Could you check a few things on this model? Use its own coordinates, in mm. Face numbers are marked on the shaded views. A direction names the side the tool comes from. Round coordinates to 2 decimals unless told otherwise and drop trailing zeros. Loops run counter-clockwise (first coordinate to the right, second up) from the corner with the lowest first, then second, coordinate; pieces in that order, holes last. Notation, with made-up numbers: (15.5, 25) - (50.5, 25) arc R26 ccw to (50.5, 43) - close; hole circle Ø6 at (0.25, 85). An arc over 180 degrees is marked (long way). Answer as CSV lines item,"result". Start each with the question number.
1) We'd pull the mould along Y, two halves only. Please class the marked faces 6, 7 and 8: pulls with the +Y half, pulls with the -Y half, needs draft (parallel to the pull), parting line crosses it, or undercut.
2) Suppose I cut it at B-B, the plane z = -155.5. Write out the boundary of the cut face in (x, y).
3) Suppose I cut it at D-D, the plane y = 74. Write out the boundary of the cut face in (x, z).
4) Suppose I cut it at A-A, the plane y = 41.5. Write out the boundary of the cut face in (x, z), then the cut area to 3 significant figures.
5) Please list where these lines run through material, in increasing order: line 1 along Z through (x, y) = (13.25, 49); line 2 along Z through (x, y) = (1.5, 51); line 3 along Z through (x, y) = (18, 42).
6) I'm going to push flat-ended pins straight in: pin 1 Ø1 at (x, y) = (7.5, 61.5) entering from -Z; pin 2 Ø10 at (x, y) = (7, 14.5) entering from +Z; pin 3 Ø2 at (x, z) = (14, -10.5) entering from +Y. Where does each tip first touch, or does it pass through?
7) Suppose I cut it at C-C, the plane y = 24. Write out the boundary of the cut face in (x, z), then the cut area to 3 significant figures.
8) Which directions (+Z, -Z, +X, -X, +Y, -Y) give clear straight access to the entire face, cutting with the end or side of a thin tool? Please do the marked faces 1, 2, 3, 4 and 5.
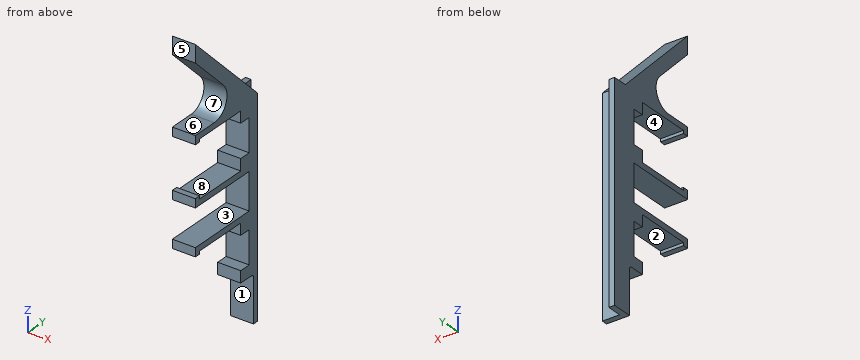
```python
from build123d import *

# Parameters (mm, degrees)
SKETCH1_W           = 5
SKETCH1_H           = 5
SKETCH1_W_2         = 35
BOSS_EXTRUDE2_DEPTH = 20
FILLET1_R           = 15
FILLET2_R           = 2
BOSS_EXTRUDE3_DEPTH = 12.7


with BuildPart() as part:
    # Sketch1 → Boss-Extrude2 (new body)
    with BuildSketch(Plane(origin=(0, 0, 0), x_dir=(0, 0, -1), z_dir=(1, 0, 0))):
        Polygon((-5, 53.5), (-5, 68.5), (-78.5, -5), (-63.5, -5), align=None)
        Polygon((69.5, 68.5), (-5, 68.5), (-5, 53.5), (-5, -5), (2.5, -5), (2.5, 0), (0, 0), (0, 48.5), (10, 48.5), (10, 58.5), (38.5, 58.5), (38.5, 48.5), (48.5, 48.5), (48.5, 0), (53.5, 0), (53.5, 58.5), (69.5, 58.5), align=None)
        Polygon((139, 68.5), (69.5, 68.5), (69.5, 58.5), (85.5, 58.5), (85.5, 0), (90.5, 0), (90.5, 48.5), (100.5, 48.5), (100.5, 58.5), (129, 58.5), (129, 48.5), (139, 48.5), (139, 63.5), align=None)
        Polygon((90.5, 0), (93, 0), (93, -5), (85.5, -5), (85.5, 0), align=None)
        Polygon((53.5, -5), (46, -5), (46, 0), (48.5, 0), (53.5, 0), align=None)
        with Locations((141.5, 66)):
            Rectangle(SKETCH1_W, SKETCH1_H)
        with Locations((161.5, 66)):
            Rectangle(SKETCH1_W_2, SKETCH1_H)
    extrude(amount=BOSS_EXTRUDE2_DEPTH)

    # Fillet1
    fillet1_edges = [part.edges().sort_by_distance(p)[0] for p in [
        (10, 53.5, 5),
    ]]
    fillet(fillet1_edges, radius=FILLET1_R)

    # Fillet2
    fillet2_edges = [part.edges().sort_by_distance(p)[0] for p in [
        (10, 63.5, -139),
    ]]
    fillet(fillet2_edges, radius=FILLET2_R)

    # Sketch2 → Boss-Extrude3 (add)
    with BuildSketch(Plane(origin=(0, 68.5, 0), x_dir=(1, 0, 0), z_dir=(0, 1, 0))):
        Polygon((5, 35), (5, 179), (0, 179), (0, -5), (5, -5), align=None)
    extrude(amount=BOSS_EXTRUDE3_DEPTH)


solid = part.part
```
Filled sheet:
1,face 6,"needs draft"
1,face 7,"pulls with the -Y half"
1,face 8,"undercut"
2,outline,"(0, 63.5) - (20, 63.5) - (20, 68.5) - (5, 68.5) - (5, 81.2) - (0, 81.2) - close"
3,outline,"(0, -179) - (5, -179) - (5, 5) - (0, 5) - close"
4,outline,"(0, -90.5) - (20, -90.5) - (20, -85.5) - (0, -85.5) - close; (0, -53.5) - (20, -53.5) - (20, -48.5) - (0, -48.5) - close; (0, 0) - (20, 0) - (20, 32) - (0, 32) - close"
4,area,"840 mm²"
5,line 1,"-139 to -129, -100.5 to -85.5, -53.5 to -38.5, -10 to 24.5"
5,line 2,"-139 to -129, -100.5 to -85.5, -53.5 to -38.5, -10 to 22.5"
5,line 3,"-90.5 to -85.5, -53.5 to -48.5, 0 to 31.5"
6,pin 1,"z = -139.06"
6,pin 2,"z = 64"
6,pin 3,"y = 68.5"
7,outline,"(0, -90.5) - (20, -90.5) - (20, -85.5) - (0, -85.5) - close; (0, -53.5) - (20, -53.5) - (20, -48.5) - (0, -48.5) - close; (0, 0) - (20, 0) - (20, 6.59) - (0, 6.59) - close; (0, 34.5) - (20, 34.5) - (20, 49.5) - (0, 49.5) - close"
7,area,"632 mm²"
8,face 1,"-Z, +X, -X, -Y"
8,face 2,"-Z, +X, -X"
8,face 3,"+X, -X, -Y"
8,face 4,"+X, -X"
8,face 5,"+Z, -Z, +X, -X, -Y"
